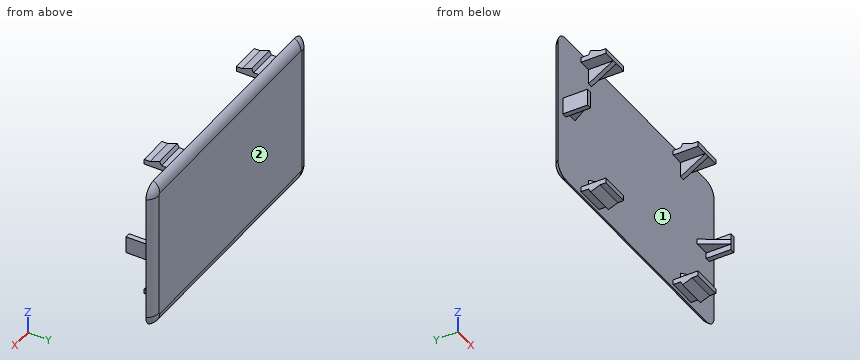
```python
from build123d import *

# Parameters (mm, degrees)
BOSS_EXTRUDE1_DEPTH  = 2.5
FILLET1_R            = 5
BOSS_EXTRUDE2_DEPTH  = 9.8
CUT_EXTRUDE1_DEPTH   = 9.8
CUT_EXTRUDE2_DEPTH   = 89.657557489
BOSS_EXTRUDE3_DEPTH  = 11.7
MIRROR4_COPY_1_DEPTH = 11.7


with BuildPart() as part:
    # Sketch1 → Boss-Extrude1 (new body)
    with BuildSketch(Plane(origin=(0, 0, 0), x_dir=(1, 0, 0), z_dir=(0, 1, 0))):
        with BuildLine():
            Line((-46.5, 30), (46.5, 30))
            ThreePointArc((46.5, 30), (50.035533906, 28.535533906), (51.5, 25))
            Line((51.5, 25), (51.5, -25))
            ThreePointArc((51.5, -25), (50.035533906, -28.535533906), (46.5, -30))
            Line((46.5, -30), (-46.5, -30))
            ThreePointArc((-46.5, -30), (-50.035533906, -28.535533906), (-51.5, -25))
            Line((-51.5, -25), (-51.5, 25))
            ThreePointArc((-51.5, 25), (-50.035533906, 28.535533906), (-46.5, 30))
        make_face()
    extrude(amount=BOSS_EXTRUDE1_DEPTH)

    # Fillet1
    # the kernel refuses this fillet: 5 mm, written as the material it takes off along each edge
    with BuildSketch(Plane(origin=(-46.5, 2.5, -25), x_dir=(-1, 0, 0), z_dir=(0, 0, 1))) as fillet1_piece_1:
        with BuildLine():
            CenterArc((0.669872981, 5), FILLET1_R, 270, 60)
            Line((0.669872981, 0), (0.669872981, -0.1))
            Line((0.669872981, -0.1), (5, -0.1))
            Line((5, -0.1), (5.1, 0))
            ThreePointArc((5.1, 0), (5.1, 1.25), (5.08660254, 2.45))
            Line((5.08660254, 2.45), (5, 2.5))
        make_face()
    revolve(axis=Axis((-46.5, 2.5, -25), (0, -1, 0)), revolution_arc=90, mode=Mode.SUBTRACT)
    with BuildSketch(Plane(origin=(-46.5, 2.5, -30), x_dir=(0, -1, 0), z_dir=(1, 0, 0)), Plane(origin=(46.5, 2.5, 30), x_dir=(0, -1, 0), z_dir=(-1, 0, 0))) as fillet1_piece_2:
        with BuildLine():
            CenterArc((5, -4.330127019), FILLET1_R, 120, 60)
            Line((0, -4.330127019), (-0.1, -4.330127019))
            Line((-0.1, -4.330127019), (-0.1, 0))
            Line((-0.1, 0), (0, 0.1))
            ThreePointArc((0, 0.1), (1.25, 0.1), (2.45, 0.08660254))
            Line((2.45, 0.08660254), (2.5, 0))
        make_face()
    extrude(amount=93, mode=Mode.SUBTRACT)
    with BuildSketch(Plane(origin=(46.5, 2.5, -25), x_dir=(0, 0, -1), z_dir=(-1, 0, 0))) as fillet1_piece_3:
        with BuildLine():
            CenterArc((0.669872981, 5), FILLET1_R, 270, 60)
            Line((0.669872981, 0), (0.669872981, -0.1))
            Line((0.669872981, -0.1), (5, -0.1))
            Line((5, -0.1), (5.1, 0))
            ThreePointArc((5.1, 0), (5.1, 1.25), (5.08660254, 2.45))
            Line((5.08660254, 2.45), (5, 2.5))
        make_face()
    revolve(axis=Axis((46.5, 2.5, -25), (0, -1, 0)), revolution_arc=90, mode=Mode.SUBTRACT)
    with BuildSketch(Plane(origin=(51.5, 2.5, -25), x_dir=(0, -1, 0), z_dir=(0, 0, 1)), Plane(origin=(-51.5, 2.5, 25), x_dir=(0, -1, 0), z_dir=(0, 0, -1))) as fillet1_piece_4:
        with BuildLine():
            CenterArc((5, -4.330127019), FILLET1_R, 120, 60)
            Line((0, -4.330127019), (-0.1, -4.330127019))
            Line((-0.1, -4.330127019), (-0.1, 0))
            Line((-0.1, 0), (0, 0.1))
            ThreePointArc((0, 0.1), (1.25, 0.1), (2.45, 0.08660254))
            Line((2.45, 0.08660254), (2.5, 0))
        make_face()
    extrude(amount=50, mode=Mode.SUBTRACT)
    with BuildSketch(Plane(origin=(46.5, 2.5, 25), x_dir=(1, 0, 0), z_dir=(0, 0, -1))) as fillet1_piece_5:
        with BuildLine():
            CenterArc((0.669872981, 5), FILLET1_R, 270, 60)
            Line((0.669872981, 0), (0.669872981, -0.1))
            Line((0.669872981, -0.1), (5, -0.1))
            Line((5, -0.1), (5.1, 0))
            ThreePointArc((5.1, 0), (5.1, 1.25), (5.08660254, 2.45))
            Line((5.08660254, 2.45), (5, 2.5))
        make_face()
    revolve(axis=Axis((46.5, 2.5, 25), (0, -1, 0)), revolution_arc=90, mode=Mode.SUBTRACT)
    with BuildSketch(Plane(origin=(-46.5, 2.5, 25), x_dir=(0, 0, 1), z_dir=(1, 0, 0))) as fillet1_piece_6:
        with BuildLine():
            CenterArc((0.669872981, 5), FILLET1_R, 270, 60)
            Line((0.669872981, 0), (0.669872981, -0.1))
            Line((0.669872981, -0.1), (5, -0.1))
            Line((5, -0.1), (5.1, 0))
            ThreePointArc((5.1, 0), (5.1, 1.25), (5.08660254, 2.45))
            Line((5.08660254, 2.45), (5, 2.5))
        make_face()
    revolve(axis=Axis((-46.5, 2.5, 25), (0, -1, 0)), revolution_arc=90, mode=Mode.SUBTRACT)

    # Sketch2 → Boss-Extrude2 (add)
    with BuildSketch(Plane.XZ):
        Polygon((-36.2, 28.5), (-24.5, 28.5), (-24.5, 26.5), (-29.35, 26.5), (-29.35, 20.5), (-31.35, 20.5), (-31.35, 26.5), (-36.2, 26.5), align=None)
        Polygon((48.225, -3.282847821), (46.225, -3.282847821), (46.225, -0.999790058), (40.225, -0.999790058), (40.225, 1), (46.225, 1), (46.225, 3.417152179), (48.225, 3.417152179), align=None)
        Polygon((24.5, 28.5), (36.2, 28.5), (36.2, 26.5), (31.35, 26.5), (31.35, 20.5), (29.35, 20.5), (29.35, 26.5), (24.5, 26.5), align=None)
        Polygon((24.5, -26.5), (29.35, -26.5), (29.35, -20.5), (31.35, -20.5), (31.35, -26.5), (36.2, -26.5), (36.2, -28.5), (24.5, -28.5), align=None)
        Polygon((-36.2, -28.5), (-24.5, -28.5), (-24.5, -26.5), (-29.35, -26.5), (-29.35, -20.5), (-31.35, -20.5), (-31.35, -26.5), (-36.2, -26.5), align=None)
        Polygon((-48.225, 3.417152179), (-46.225, 3.417152179), (-46.225, 1), (-40.225, 1), (-40.225, -0.999790058), (-46.225, -0.999790058), (-46.225, -3.282847821), (-48.225, -3.282847821), align=None)
    extrude(amount=BOSS_EXTRUDE2_DEPTH)

    # Sketch4 → Cut-Extrude1 (cut)
    with BuildSketch(Plane(origin=(0, 0, -0.999790058), x_dir=(-1, 0, 0), z_dir=(0, 0, -1))):
        Polygon((40.225, 0), (46.225, -9.8), (40.225, -9.8), align=None)
    cut_extrude1 = extrude(amount=-CUT_EXTRUDE1_DEPTH, mode=Mode.SUBTRACT)

    # Mirror1: Cut-Extrude1 across plane
    add(cut_extrude1.mirror(Plane(origin=(0, 0, 0), x_dir=(0, 0, 1), z_dir=(1, 0, 0))), mode=Mode.SUBTRACT)

    # Sketch5 → Cut-Extrude2 (cut, through all)
    with BuildSketch(Plane.ZY.offset(31.35)):
        Polygon((-26.5, -9.8), (-20.5, 0), (-20.5, -9.8), align=None)
    cut_extrude2 = extrude(amount=-CUT_EXTRUDE2_DEPTH, mode=Mode.SUBTRACT)

    # Mirror2: Cut-Extrude2 across plane
    add(cut_extrude2.mirror(Plane.XY), mode=Mode.SUBTRACT)

    # Sketch6 → Boss-Extrude3 (add)
    with BuildSketch(Plane(origin=(36.2, 0, 0), x_dir=(0, 0, -1), z_dir=(1, 0, 0))):
        Polygon((-28.5, -3), (-28.5, -7.5), (-30, -3.726144837), align=None)
    boss_extrude3 = extrude(amount=-BOSS_EXTRUDE3_DEPTH)

    # Mirror3: Boss-Extrude3 across plane
    add(boss_extrude3.mirror(Plane(origin=(0, 0, 0), x_dir=(0, 0, 1), z_dir=(1, 0, 0))))

    # Mirror4: Boss-Extrude3 across plane
    add(boss_extrude3.mirror(Plane.XY))

    # Mirror4 copy 1 sketch → Mirror4 copy 1 (add)
    with BuildSketch(Plane.ZY.offset(36.2)):
        Polygon((-28.5, -3), (-28.5, -7.5), (-30, -3.726144837), align=None)
    extrude(amount=-MIRROR4_COPY_1_DEPTH)


solid = part.part
```
Source: CAD feature listing. Evaluate the final solid. Frame: model axes, mm. Face numbers are marked on the shaded views. Round coordinates to 2 decimals unless told otherwise and drop trailing zeros. Order: outer loops, then holes, each group sorted by start corner. A loop starts at its lowest first (then second) coordinate and runs counter-clockwise, first axis right, second up. Notation, with made-up numbers: (10.25, 14.25) -> (52.25, 14.25) arc R4 ccw to (52.25, 21.25) -> close; hole circle Ø10 at (28, 16.25). An arc over 180 degrees is marked (long way). One line per item, written item: value. Start each with the question number.
Q1. Section query C-C (z = 19). Return the cut outline in (x, y).
Q2. Draft query along X for the marked faces 1 and 2. Return one class per face: pulls with the +X half, pulls with the -X half, needs draft (parallel to the pull), parting line crosses it, or undercut.
Q3. Pin query (flat end, axial travel): pin 1 (5 mm diameter, centred on x = 31.5, z = 16.5, fed in from -Y); pin 2 (5 mm diameter, centred on x = 44, y = -4.5, fed in from -Z); pin 3 (1.6 mm diameter, centred on x = -47.5, y = -4.5, fed in from +Z). Return the tip coordinate at first contact, or that it passes through.
Q4. Section query B-B (y = -2). Give the number of separate pieces and of enclosed holes in the cut face, plus the area to 3 significant figures.
Q5. Material intervals for probe 1 along X at (y, z) = (-3, -1.5) (3 decimals); probe 2 along X at (y, z) = (-2.5, -25); probe 3 along Z at (x, y) = (-27, -6.75), sorted ascending.
Q6. Section query A-A (x = -33). Return the cut outline in (y, z), plus the area to 3 significant figures.
Q7. Section query D-D (x = 15). Return the cut outline in (y, z), plus the area to 3 significant figures.
Findings below:
1. outline: (-51.5, 0) -> (51.5, 0) arc R5 ccw to (47.17, 2.5) -> (-47.17, 2.5) arc R5 ccw to start
2. face 1: undercut
2. face 2: needs draft
3. pin 1: y = 0
3. pin 2: z = -3.28
3. pin 3: z = 3.42
4. separate pieces: 6
4. enclosed holes: 0
4. area: 178 mm²
5. probe 1: -48.225 to -46.225, 46.225 to 48.225
5. probe 2: -31.35 to -29.35, 29.35 to 31.35
5. probe 3: -28.8 to -26.5, 26.5 to 28.8
6. outline: (-9.8, -28.5) -> (-7.5, -28.5) -> (-3.73, -30) -> (-3, -28.5) -> (0, -28.5) -> (0, -30) arc R5 ccw to (2.5, -25.67) -> (2.5, 25.67) arc R5 ccw to (0, 30) -> (0, 28.5) -> (-3, 28.5) -> (-3.73, 30) -> (-7.5, 28.5) -> (-9.8, 28.5) -> (-9.8, 26.5) -> (0, 26.5) -> (0, -26.5) -> (-9.8, -26.5) -> close
6. area: 190 mm²
7. outline: (0, -30) arc R5 ccw to (2.5, -25.67) -> (2.5, 25.67) arc R5 ccw to (0, 30) -> close
7. area: 144 mm²
